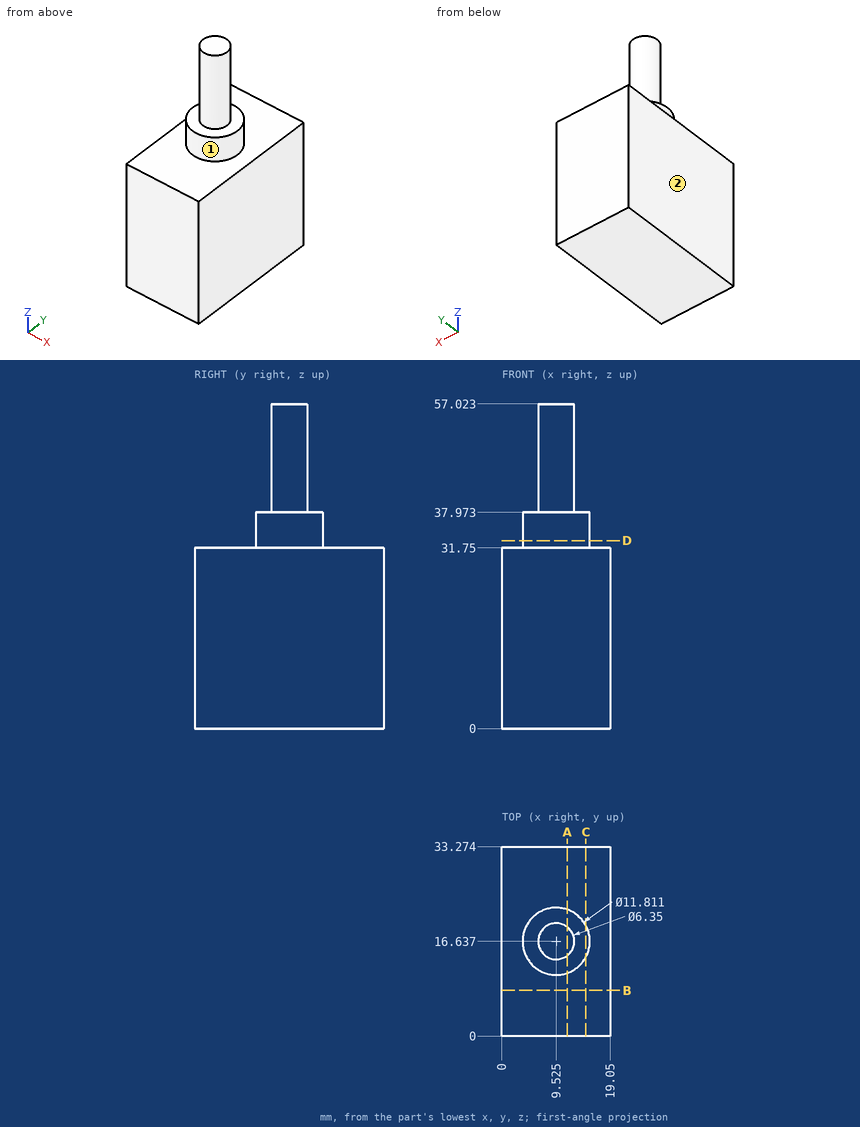
Study the drawing (mm; zero at the part's minimum x, y, z) and answer. A direction names the side the tool comes from. Coordinates: 2 decimals unless noted, no trailing zeros. Loops run counter-clockwise (first coordinate to the right, second up) from the corner with the lowest first, then second, coordinate; pieces in that order, holes last. Notation, with made-up numbers: (63.5, 21.25) -> (80.5, 21.25) arc R23 ccw to (80.5, 32.25) -> close; hole circle Ø9 at (42.5, 89). An arc over 180 degrees is marked (long way). Answer as CSV lines item,"result".
1) The part is cut by section D-D (z = 33). Give the vertices of the cut face in (x, y) (1 decimal).
A:
outline,"circle Ø11.8 at (9.5, 16.6)"
2) The part is cut by section C-C (x = 14.75). Give the vertices of the cut face in (y, z), and give its area (3 significant figures).
A:
outline,"(0, 0) -> (33.27, 0) -> (33.27, 31.75) -> (19.39, 31.75) -> (19.39, 37.97) -> (13.88, 37.97) -> (13.88, 31.75) -> (0, 31.75) -> close"
area,"1,090 mm²"
3) For the marked faces 1 and 2, determine the directions among +Z, -Z, +X, -X, +Y, -Y from which every point of the face is accessible in a straight line to the end or side of a thin tool.
A:
face 1,"+Z"
face 2,"+Z, -Z, -X, +Y, -Y"
4) Straight lines are drawn through the part: probe 1 along Z at (x, y) = (12.5, 12); probe 2 along Z at (x, y) = (8.5, 22.5); probe 3 along X at (y, z) = (16, 37.5). For each, find the intervals that lie inside material, in ascending order.
A:
probe 1,"z = 0 to 37.97"
probe 2,"z = 0 to 31.75"
probe 3,"x = 3.65 to 15.4"
5) The part is cut by section B-B (y = 8). Give the vertices of the cut face in (x, z).
A:
outline,"(0, 0) -> (19.05, 0) -> (19.05, 31.75) -> (0, 31.75) -> close"
6) Flat-ended cylindrical pins translate along their axes: pin 1 (4 mm diameter, centred on x = 7, z = 39.5, fed in from -Y); pin 2 (6 mm diameter, centred on x = 2, y = 4, fed in from +Z). Find the tip coordinate at first contact, or state that the pin passes through.
A:
pin 1,"stops at y = 10.86"
pin 2,"stops at z = 31.75"
7) The part is cut by section A-A (x = 11.5). Give the vertices of the cut face in (y, z).
A:
outline,"(0, 0) -> (33.27, 0) -> (33.27, 31.75) -> (22.2, 31.75) -> (22.2, 37.97) -> (19.12, 37.97) -> (19.12, 57.02) -> (14.15, 57.02) -> (14.15, 37.97) -> (11.07, 37.97) -> (11.07, 31.75) -> (0, 31.75) -> close"
